Source: CAD feature listing. Evaluate the final solid. Frame: model axes, mm. Coordinates: 2 decimals unless noted, no trailing zeros. Order: outer loops, then holes, each group sorted by start corner. A loop starts at its lowest first (then second) coordinate and runs counter-clockwise, first axis right, second up. Notation, with made-up numbers: (-37, 80) - (0, 80) arc R33 ccw to (0, 111) - close; hole circle Ø6 at (4.5, 23.25). An arc over 180 degrees is marked (long way). One line per question, with ' | ' between items.
from build123d import *

# Parameters (mm, degrees)
F1_DEPTH = 3.81


with BuildPart() as f1:
    # F0 (on Front) → F1 (new body)
    with BuildSketch(Plane.XZ):
        Polygon((-56.769, 0), (-56.769, -25.908), (56.769, -25.908), (56.769, 0), (56.769, 25.908), (-56.769, 25.908), align=None)
        with BuildLine():
            ThreePointArc((-14.859, 0), (-34.671, -19.812), (-54.483, 0))
            ThreePointArc((-54.483, 0), (-34.671, 19.812), (-14.859, 0))
        make_face(mode=Mode.SUBTRACT)
        with BuildLine():
            ThreePointArc((10.795, 0), (30.607, 19.812), (50.419, 0))
            ThreePointArc((50.419, 0), (30.607, -19.812), (10.795, 0))
        make_face(mode=Mode.SUBTRACT)
    extrude(amount=F1_DEPTH)


solid = f1.part
(1) Cut plane D-D (z = 10). Return the cut outline in (x, y), and give its area (3 significant figures).
Taken from the geometry:
outline: (-56.77, -3.81) - (-51.77, -3.81) - (-51.77, 0) - (-56.77, 0) - close; (-17.57, -3.81) - (13.5, -3.81) - (13.5, 0) - (-17.57, 0) - close; (47.71, -3.81) - (56.77, -3.81) - (56.77, 0) - (47.71, 0) - close | area: 172 mm²
(2) Material intervals for L1, parallel to X at y = -1.9, z = 8.5; L2, parallel to X at y = -2.95, z = -2; L3, parallel to Z at x = -19, y = -2.8, sorted ascending. Write a range as from..to.
Taken from the geometry:
L1: x = -56.77..-52.57, -16.78..12.71, 48.5..56.77 | L2: x = -56.77..-54.38, -14.96..10.9, 50.32..56.77 | L3: z = -25.91..-12.12, 12.12..25.91
(3) Pull-direction query (Z, two-part tool) for faces 1 (the flat face through (1, -2, 25.908)), 2 (the flat face through (-1, 0, 0)), 3 (the cylindrical face through (49.504, -1.878, -5.951)); classes: pulls with the +Z half, pulls with the -Z half, needs draft (parallel to the pull), parting line crosses it, or undercut.
Taken from the geometry:
face 1: pulls with the +Z half | face 2: needs draft | face 3: undercut
(4) Cut plane A-A (z = 0). Return the cut outline in (x, y) (3 decimals).
Taken from the geometry:
outline: (-56.769, -3.81) - (-54.483, -3.81) - (-54.483, 0) - (-56.769, 0) - close; (-14.859, -3.81) - (10.795, -3.81) - (10.795, 0) - (-14.859, 0) - close; (50.419, -3.81) - (56.769, -3.81) - (56.769, 0) - (50.419, 0) - close
(5) Cut plane C-C (y = -2.8). Return the cut outline in (x, z), and give its area (3 significant figures).
Taken from the geometry:
outline: (-56.77, -25.91) - (56.77, -25.91) - (56.77, 25.91) - (-56.77, 25.91) - close; hole circle Ø39.62 at (-34.67, 0); hole circle Ø39.62 at (30.61, 0) | area: 3,420 mm²
(6) Pin query (flat end, axial travel): P1, Ø8, axis at x = -8.5, z = -17, coming from the +Y side; P2, Ø24, axis at x = 30.607, z = 0, coming from the +Y side. Return the tip coordinate at first contact, or that it passes through.
Taken from the geometry:
P1: stops at y = 0 | P2: passes through
(7) Cut plane B-B (x = -45.5). Return the cut outline in (y, z).
Taken from the geometry:
outline: (-3.81, -25.91) - (0, -25.91) - (0, -16.59) - (-3.81, -16.59) - close; (-3.81, 16.59) - (0, 16.59) - (0, 25.91) - (-3.81, 25.91) - close
